Geometry: final body of the model. Coordinates: model frame, mm. Round coordinates to 2 decimals unless told otherwise and drop trailing zeros. Order: outer loops, then holes, each group sorted by start corner. A loop starts at its lowest first (then second) coordinate and runs counter-clockwise, first axis right, second up. Notation, with made-up numbers: M -30.5,70 L 12.5,70 A12 ccw 12.5,93 Z; hole C -26,-4 d8. An arc over 180 degrees is marked long. Put each result on its own line as item: value. Start each with the question number.
1) Section D-D, the plane z = -281.5. Return loops of the section in (x, y) (3 decimals).
2) Draft query along Y for faces 1 (the flat face through (0, 615, -460)), 2 (the cylindrical face through (1.61, 300.044, -337.129)), 3 (the flat face through (1.6, 1184.3, -173.7)). Return one class per face: pulls with the +Y half, pulls with the -Y half, needs draft (parallel to the pull), parting line crosses it, or undercut.
3) Material intervals for probe 1 along Y at (x, z) = (1.3, -44.45); probe 2 along Y at (x, z) = (2.05, -631.5); probe 3 along Y at (x, z) = (0.9, -152.4), sorted ascending. Write a range as [from, to].
4) Section A-A, the plane y = 307.34. Return loops of the section in (x, z) (3 decimals).
5) Section B-B, the plane x = 1.6. Count the separate pieces of the cut face and the enclosed holes in it, then the cut area to 3 significant figures.
6) Section C-C, the plane z = -837.5. Return loops of the section in (x, y) (3 decimals), then the cut area to 3 significant figures.
7) First-contact query: P1, Ø6.5, axis at y = 69.85, z = -44.45, coming from the +X side. Flat tip, straight axial feed; report the tip coordinate or a pass-through.
from build123d import *

# Parameters (mm, degrees)
BOSS_EXTRUDE1_DEPTH            = 3.175
SKETCH2_R                      = 19.05
CUT_EXTRUDE1_DEPTH             = 4.175
FILLET1_R                      = 6.35
F_5_16_0_3125_DIAMETER_HOLE1_D = 7.9375


with BuildPart() as part:
    # Sketch1 → Boss-Extrude1 (new body)
    with BuildSketch(Plane(origin=(0, 0, 0), x_dir=(0, 0, -1), z_dir=(1, 0, 0))):
        Polygon((0, 0), (933.45, 0), (933.45, 1089.025), (342.9, 1193.154898457), (342.9, 1154.467144545), (0, 1214.929666229), align=None)
    extrude(amount=BOSS_EXTRUDE1_DEPTH)

    # Sketch2 → Cut-Extrude1 (cut, through all)
    with BuildSketch(Plane(origin=(3.175, 0, 0), x_dir=(0, 0, -1), z_dir=(1, 0, 0))):
        with Locations((319.532, 307.34)):
            Circle(SKETCH2_R)
    extrude(amount=-CUT_EXTRUDE1_DEPTH, mode=Mode.SUBTRACT)

    # Fillet1
    fillet1_edges = [part.edges().sort_by_distance(p)[0] for p in [
        (1.5875, 1214.929666229, 0),
        (1.5875, 1154.467144545, -342.9),
        (1.5875, 1193.154898457, -342.9),
        (1.5875, 1089.025, -933.45),
        (1.5875, 0, -933.45),
        (1.5875, 0, 0),
    ]]
    fillet(fillet1_edges, radius=FILLET1_R)

    # 5/16 (0.3125) Diameter Hole1 (through all)
    with Locations(Plane(origin=(3.175, 0, 0), x_dir=(0, 0, -1), z_dir=(1, 0, 0))):
        with Locations((44.45, 1149.35), (44.45, 635), (152.4, 330.2), (152.4, 282.575), (635, 330.2), (635, 282.575), (892.175, 517.525), (892.175, 1028.7), (374.65, 1148.868762907), (793.75, 1074.970125292), (44.45, 69.85)):
            Hole(F_5_16_0_3125_DIAMETER_HOLE1_D / 2)


solid = part.part
Result sheet:
1. outline: M 0,0 L 3.175,0 L 3.175,1165.294 L 0,1165.294 Z
2. face 1: needs draft
2. face 2: undercut
2. face 3: pulls with the +Y half
3. probe 1: y = [0, 65.88], [73.82, 631.03], [638.97, 1145.38], [1153.32, 1207.09]
3. probe 2: y = [0, 280.7], [284.45, 328.33], [332.07, 1142.27]
3. probe 3: y = [0, 278.61], [286.54, 326.23], [334.17, 1188.06]
4. outline: M 0,-933.45 L 3.175,-933.45 L 3.175,-338.582 L 0,-338.582 Z; M 0,-300.482 L 3.175,-300.482 L 3.175,0 L 0,0 Z
5. separate pieces: 1
5. enclosed holes: 12
5. area: 1,080,000 mm2
6. outline: M 0,0 L 3.175,0 L 3.175,1105.944 L 0,1105.944 Z
6. area: 3,510 mm2
7. P1: passes through
